Can you work these out from the model? Positions are in its coordinate system, mm. A direction names the side the tool comes from. Give positions to 0.01 mm unless a question says otherwise; leave off trailing zeros. Loops run counter-clockwise (first coordinate to the right, second up) from the corner with the lowest first, then second, coordinate; pieces in that order, holes last. Notation, with made-up numbers: (23, -4) - (57, -4) arc R9 ccw to (57, 2) - close; hole circle Ø1 at (-35, 64.25). An arc over 180 degrees is marked (long way). Answer in a Markdown table with one row per item.
from build123d import *

# Parameters (mm, degrees)
CROQUIS1_R                   = 5
CROQUIS1_R_2                 = 12
SALIENTE_EXTRUIR1_DEPTH      = 3
TALADRO_DE_MARGEN_PARA_M32_D = 3.4
TALADRO_ROSCADO_M3X0_51_D    = 2.5
CROQUIS8_W                   = 6
CROQUIS8_H                   = 15
CORTAR_EXTRUIR1_DEPTH        = 75.491610266
CROQUIS9_W                   = 15
CROQUIS9_H                   = 6
SALIENTE_EXTRUIR3_DEPTH      = 6


with BuildPart() as part:
    # Croquis1 → Saliente-Extruir1 (new, symmetric)
    with BuildSketch(Plane(origin=(0, 0, 0), x_dir=(0, 0, -1), z_dir=(1, 0, 0))):
        with BuildLine():
            Line((-32, -35), (-32, 35))
            ThreePointArc((-32, 35), (0, 67), (32, 35))
            Line((32, 35), (32, -35))
            Line((32, -35), (-32, -35))
        make_face()
        with Locations((0, 35)):
            Circle(CROQUIS1_R, mode=Mode.SUBTRACT)
        with Locations((0, -11)):
            Circle(CROQUIS1_R_2, mode=Mode.SUBTRACT)
    extrude(amount=SALIENTE_EXTRUIR1_DEPTH, both=True)

    # Taladro de margen para M32 (through all)
    with Locations(Plane(origin=(3, 0, 0), x_dir=(0, 0, -1), z_dir=(1, 0, 0))):
        with Locations((-15.5, 4.5), (-15.5, -26.5), (15.5, -26.5), (15.5, 4.5)):
            Hole(TALADRO_DE_MARGEN_PARA_M32_D / 2)

    # Taladro roscado M3x0.51 (through all)
    with Locations(Plane.ZY.offset(3)):
        with Locations((-12.5, 22.5), (-12.5, 47.5), (12.5, 47.5), (12.5, 22.5)):
            Hole(TALADRO_ROSCADO_M3X0_51_D / 2)

    # Croquis8 → Cortar-Extruir1 (cut, through all)
    with BuildSketch(Plane(origin=(3, 0, 0), x_dir=(0, 0, -1), z_dir=(1, 0, 0))):
        with Locations((-25, 2.5)):
            Rectangle(CROQUIS8_W, CROQUIS8_H)
        with Locations((-25, -27.5)):
            Rectangle(CROQUIS8_W, CROQUIS8_H)
        with Locations((25, -27.5)):
            Rectangle(CROQUIS8_W, CROQUIS8_H)
        with Locations((25, 2.5)):
            Rectangle(CROQUIS8_W, CROQUIS8_H)
    extrude(amount=-CORTAR_EXTRUIR1_DEPTH, mode=Mode.SUBTRACT)

    # Croquis9 → Saliente-Extruir3 (add, through all)
    with BuildSketch(Plane(origin=(3, 0, 0), x_dir=(0, 0, -1), z_dir=(1, 0, 0))):
        with Locations((-12.5, -38)):
            Rectangle(CROQUIS9_W, CROQUIS9_H)
        with Locations((12.5, -38)):
            Rectangle(CROQUIS9_W, CROQUIS9_H)
    extrude(amount=-SALIENTE_EXTRUIR3_DEPTH)


solid = part.part
Q1. For pin 1 (1.8 mm diameter, centred on x = 0, y = -39.5, fed in from +Z); pin 2 (3 mm diameter, centred on x = 1, z = 25, fed in from -Y); pin 3 (3 mm diameter, centred on x = 0, y = -37, fed in from -Z), each with a flat end and sliding along its axis, tell me the tip position at first contact or that it passes through.
Checked values:
| item | result |
|---|---|
| pin 1 | stops at z = 20 |
| pin 2 | stops at y = -20 |
| pin 3 | stops at z = -20 |
Q2. Imagine slicing it at D-D, the plane x = -0.65. Count the separate pieces of the cut face and the enclosed holes in it, and give its area (3 significant figures).
Checked values:
| item | result |
|---|---|
| separate pieces | 1 |
| enclosed holes | 12 |
| area | 5,320 mm² |
Q3. Imagine slicing it at B-B, the plane y = -11. Write out the boundary of the cut face in (x, z).
Checked values:
| item | result |
|---|---|
| outline | (-3, -32) - (3, -32) - (3, -12) - (-3, -12) - close; (-3, 12) - (3, 12) - (3, 32) - (-3, 32) - close |
Q4. Imagine slicing it at C-C, the plane y = 22.5. Write out the boundary of the cut face in (x, z).
Checked values:
| item | result |
|---|---|
| outline | (-3, -32) - (3, -32) - (3, -13.75) - (-3, -13.75) - close; (-3, -11.25) - (3, -11.25) - (3, 11.25) - (-3, 11.25) - close; (-3, 13.75) - (3, 13.75) - (3, 32) - (-3, 32) - close |
Q5. On a 3-axis mill with a long thin cutter (end or side, diameter ignored), from which of +Z, -Z, +X, -X, +Y, -Y can I reach the whole of each face in a straight line? I mean faces 4 (the face through (0, 2, -28)), 5 (the face through (0, -35, 21)), 6 (the face through (0, -20, 25)), 7 (the face through (0, -35, -30)). Say none if no direction works.
Checked values:
| item | result |
|---|---|
| face 4 | +X, -X |
| face 5 | +Z, +X, -X, -Y |
| face 6 | +X, -X, -Y |
| face 7 | -Z, +X, -X, -Y |
Q6. If I drill on line 1 (Y direction, x = -1.5, z = -0.5); line 2 (Z direction, x = 2.05, y = -37); line 3 (Y direction, x = 0, z = 15.5), over which ranges is the centre line in solid material (lowest first)? Write a range as [from, to].
Checked values:
| item | result |
|---|---|
| line 1 | y = [-35, -22.99], [0.99, 30.03], [39.97, 67] |
| line 2 | z = [-20, -5], [5, 20] |
| line 3 | y = [-41, -28.2], [-24.8, 2.8], [6.2, 63] |
Q7. If we mould it in two halves opening along Y, with no side actions, what happens to faces 1 (the face through (0, 10, 25)), 2 (the face through (0, -41, -12)), 3 (the face through (0, -28, -22))? For each: released by +Y, released by -Y, zero draft, split by the parting line, or undercut.
Checked values:
| item | result |
|---|---|
| face 1 | undercut |
| face 2 | released by -Y |
| face 3 | zero draft |
Q8. Imagine slicing it at A-A, the plane z = 0. Write out the boundary of the cut face in (x, y).
Checked values:
| item | result |
|---|---|
| outline | (-3, -35) - (3, -35) - (3, -23) - (-3, -23) - close; (-3, 1) - (3, 1) - (3, 30) - (-3, 30) - close; (-3, 40) - (3, 40) - (3, 67) - (-3, 67) - close |
